Geometry check sheet. Reference: the model listing, model coordinates, mm. Give positions to 0.01 mm unless a question says otherwise; leave off trailing zeros. Write each loop counter-clockwise with the first axis right and the second up, starting at its lowest first coordinate (ties: lowest second). Pieces come first, ordered by that corner, then holes.
(1) Mould release check, pull along Y, two halves, no side actions. Record for faces 1 (the flat face through (-4, 291, 9)), 2 (the cylindrical face through (-87.86, 207.815, 8.874)), 3 (the flat face through (-291, -4, 9)): +Y half, -Y half, draft (parallel to the pull), parting line (faces both ways), or undercut.
(2) Depth check by flat-ended pin: P1, Ø6, axis at x = -77, z = 11, coming from the -Y side; P2, Ø1, axis at y = -24.5, z = 7.5, coming from the -X side; P3, Ø8, axis at x = -217, y = -151.5, coming from the -Z side; P4, Ø1.5, axis at y = -159.5, z = 7, coming from the +X side. Enter the tip coordinate at first touch or a pass-through.
(3) Thickness scan on line 1 along X through (y, z) = (1.5, 2.5); line 2 along X through (y, z) = (112, 9.5); line 3 along Y through (x, z) = (0, 8.75). Record the ranges inside material, lowest first.
(4) Cross-section at C-C (z = 9.75). Record the boundary of the cut face in (x, y), and give its area (3 significant figures).
Solid Edge part; units mm, degrees
sketch "Sketch1" plane through (0, 0, 0) normal (0, 0, 1) x (1, 0, 0)
  line L0 (-300, -300) -> (300, -300)
  line L1 (300, -300) -> (300, 300)
  line L2 (300, 300) -> (-300, 300)
  line L3 (-300, 300) -> (-300, -300)
extrude "Protrusion1" add sketch "Sketch1" along normal blind 18
chamfer "Chamfer_2" distance 18 angle 45 4 edges at (0, -300, 18) (300, 0, 18) (0, 300, 18) (-300, 0, 18)
sketch "Sketch2" plane through (0, 0, 0) normal (0, 0, -1) x (0, -1, 0)
  circle A0 centre (-112, 0) radius 130
extrude "ExtrudedCutout_1" cut sketch "Sketch2" against normal blind 18
properties material "Wood, Mahogany"
Reply:
1. face 1: +Y half
1. face 2: undercut
1. face 3: draft
2. P1: stops at y = -292
2. P2: stops at x = -293
2. P3: stops at z = 0
2. P4: stops at x = 293.75
3. line 1: x = -297.5 to -68.48, 68.48 to 297.5
3. line 2: x = -290.5 to -130, 130 to 290.5
3. line 3: y = -291.25 to -18, 242 to 291.25
4. outline: (-290.25, -290.25) - (290.25, -290.25) - (290.25, 290.25) - (-290.25, 290.25) - close; hole circle Ø260 at (0, 112)
4. area: 284,000 mm2
